Check sheet for the modelled part. Datum: model origin and axes. Units: mm. A direction names the side the tool comes from. Round coordinates to 2 decimals unless told otherwise and drop trailing zeros. Write each loop counter-clockwise with the first axis right and the second up, starting at its lowest first coordinate (ties: lowest second). Pieces come first, ordered by that corner, then holes. Notation, with made-up numbers: (73.5, -26) - (131.5, -26) arc R5 cw to (131.5, -21) - close; hole circle Ø8 at (-18, -36). An arc over 180 degrees is marked (long way). Use one line per item in the form item = value. Start each with the question number.
1) Set-up check for faces 4 (the face through (0, 2, -29)), 5 (the face through (-9.525, 2, 5)): record each of +Z, -Z, +X, -X, +Y, -Y from which the full face is reachable in a straight line by a thin tool's end or side.
2) Draft check along Z on faces 1 (the face through (0, 2, 9.652)), 2 (the face through (-9, 0, 8)), 3 (the face through (0, 2, -38.1)). Enter one of: +Z half, -Z half, draft (parallel to the pull), parting line (faces both ways), or undercut.
3) Section check A-A (z = 3.28). Record the boundary of the cut face in (x, y) (1 decimal).
4) Section check D-D (z = -19). Record the boundary of the cut face in (x, y) (1 decimal), then the cut area to 3 significant figures.
5) Scan lines: probe 1 along Z at (x, y) = (0, 1.1); probe 2 along X at (y, z) = (2.55, -5.5) (1 decimal); probe 3 along Z at (x, y) = (-6, 0.7). Record each from-to range of solid material in increasing order.
6) Section check B-B (x = 0). Count the separate pieces of the cut face and the enclosed holes in it, then the cut area to 3 significant figures.
from build123d import *

# Parameters (mm, degrees)
SKETCH1_W           = 19.05
SKETCH1_H           = 76.2
SKETCH1_R           = 1.5875
SKETCH1_W_2         = 13.335
SKETCH1_H_2         = 29
SKETCH1_W_3         = 12.827
SKETCH1_H_3         = 3.302
BOSS_EXTRUDE1_DEPTH = 3.175
FILLET1_R           = 8.89
FILLET2_R           = 8.89


with BuildPart() as part:
    # Sketch1 → Boss-Extrude1 (new body)
    with BuildSketch(Plane(origin=(0, 0, 0), x_dir=(1, 0, 0), z_dir=(0, 1, 0))):
        Rectangle(SKETCH1_W, SKETCH1_H)
        with Locations((0, 32.28)):
            Circle(SKETCH1_R, mode=Mode.SUBTRACT)
        with Locations((0, -3.28)):
            Circle(SKETCH1_R, mode=Mode.SUBTRACT)
        with Locations((0, 14.5)):
            Rectangle(SKETCH1_W_2, SKETCH1_H_2, mode=Mode.SUBTRACT)
        with Locations((0, -8.001)):
            Rectangle(SKETCH1_W_3, SKETCH1_H_3, mode=Mode.SUBTRACT)
    extrude(amount=BOSS_EXTRUDE1_DEPTH)

    # Fillet1
    fillet1_edges = [part.edges().sort_by_distance(p)[0] for p in [
        (9.525, 1.5875, -38.1),
    ]]
    fillet(fillet1_edges, radius=FILLET1_R)

    # Fillet2
    fillet2_edges = [part.edges().sort_by_distance(p)[0] for p in [
        (-9.525, 1.5875, -38.1),
    ]]
    fillet(fillet2_edges, radius=FILLET2_R)


solid = part.part
Results are:
q1.face_4 = +Y, -Y
q1.face_5 = +Z, -Z, -X, +Y, -Y
q2.face_1 = undercut
q2.face_2 = draft
q2.face_3 = -Z half
q3.outline = (-9.5, 0) - (-1.6, 0) - (-1.6, 3.2) - (-9.5, 3.2) - close; (1.6, 0) - (9.5, 0) - (9.5, 3.2) - (1.6, 3.2) - close
q4.outline = (-9.5, 0) - (-6.7, 0) - (-6.7, 3.2) - (-9.5, 3.2) - close; (6.7, 0) - (9.5, 0) - (9.5, 3.2) - (6.7, 3.2) - close
q4.area = 18.1 mm²
q5.probe_1 = -38.1 to -33.87, -30.69 to -29, 0 to 1.69, 4.87 to 6.35, 9.65 to 38.1
q5.probe_2 = -9.5 to -6.7, 6.7 to 9.5
q5.probe_3 = -36.3 to -29, 0 to 6.35, 9.65 to 38.1
q6.separate_pieces = 5
q6.enclosed_holes = 0
q6.area = 119 mm²
